Could you check a few things on this model? Use its own coordinates, in mm. A direction names the side the tool comes from. Give positions to 0.01 mm unless a question says otherwise; leave off trailing zeros. Order: outer loops, then holes, each group sorted by start corner. A loop starts at its lowest first (then second) coordinate and runs counter-clockwise, first axis right, second up. Notation, with made-up numbers: (16.25, 74) -> (58.25, 74) arc R21 ccw to (58.25, 107) -> close; hole circle Ø1 at (17.25, -15.5). An arc over 180 degrees is marked (long way). Write each question's results on one line, items separated by ' | '.
```python
from build123d import *

# Parameters (mm, degrees)
SKETCH3_R          = 1.4478
CUT_EXTRUDE1_DEPTH = 1.016
FILLET1_R          = 0.508
FILLET3_R          = 0.762


with BuildPart() as part:
    # Sketch2 → Revolve1 (revolve)
    with BuildSketch(Plane.XY):
        with BuildLine():
            Line((0, 0), (-4.7625, 0))
            Line((-4.7625, 0), (-4.7625, 0.254))
            ThreePointArc((-4.7625, 0.254), (-3.827073968, 1.183884704), (-2.5527, 1.524))
            Line((-2.5527, 1.524), (0, 1.524))
            Line((0, 1.524), (0, 0))
        make_face()
    revolve(axis=Axis((0, -4.155418325, 0), (0, 1, 0)))

    # Sketch3 → Cut-Extrude1 (cut)
    with BuildSketch(Plane(origin=(0, 1.524, 0), x_dir=(1, 0, 0), z_dir=(0, 1, 0))):
        Circle(SKETCH3_R)
    extrude(amount=-CUT_EXTRUDE1_DEPTH, mode=Mode.SUBTRACT)

    # Fillet1
    fillet1_edges = [part.edges().sort_by_distance(p)[0] for p in [
        (-1.4478, 1.524, 0),
    ]]
    fillet(fillet1_edges, radius=FILLET1_R)

    # Sketch5 → Revolve3 (revolve)
    with BuildSketch(Plane.XY):
        Polygon((0, 0), (-2.38125, 0), (-2.38125, -4.7625), (-3.175, -4.7625), (-3.175, -7.9375), (-1.4478, -7.9375), (-1.4478, -5.3975), (0, -5.3975), align=None)
    revolve(axis=Axis((0, 0, 0), (0, 1, 0)))

    # Fillet3
    fillet3_edges = [part.edges().sort_by_distance(p)[0] for p in [
        (3.175, -7.9375, 0),
    ]]
    fillet(fillet3_edges, radius=FILLET3_R)


solid = part.part
```
Q1. I'm going to push flat-ended pins straight in: pin 1 Ø3 at (x, y) = (2, -7) entering from -Z; pin 2 Ø5 at (x, y) = (-2.5, -6) entering from +Z (3 decimals); pin 3 Ø2 at (y, z) = (-5, 2) entering from -X; pin 4 Ø1.5 at (x, y) = (-3.5, -2) entering from +Z. Where does each tip first touch, or does it pass through?
Here are the results:
pin 1: stops at z = -3.14 | pin 2: stops at z = 3.175 | pin 3: stops at x = -3.01 | pin 4: passes through
Q2. Thinking about a two-plate mould opening in Z: for faces 5 (the cylindrical face through (0.314, -6.65, -1.413)), 6 (the cylindrical face through (1.89, -2.41, -1.45)), 7 (the cylindrical face through (-0.314, 0.766, 1.413)), 8 (the flat face through (0, -7.938, -2)), which applies, +Z half, -Z half, draft (parallel to the pull), parting line (faces both ways), or undercut?
Here are the results:
face 5: undercut | face 6: parting line | face 7: undercut | face 8: draft
Q3. For faces 1 (the flat face through (1, 1.524, -2)), 2 (the flat face through (0, 0.508, 0)), 3 (the flat face through (0, -5.398, 0)), 4 (the flat face through (2, 0, -2)), which set-ups out of +Z, -Z, +X, -X, +Y, -Y let a thin tool reach every point of the face, with its end or its side?
Here are the results:
face 1: +Z, -Z, +X, -X, +Y | face 2: +Y | face 3: -Y | face 4: none
Q4. Suppose I cut it at A-A on y = -4.5. Please give me the cut outline in (x, z), and give its area (3 significant figures).
Here are the results:
outline: circle Ø4.76 at (0, 0) | area: 17.8 mm²
Q5. I need wall thicknesses on line 1 along Z through (x, y) = (0, -6.7) (3 decimals); line 2 along Z through (x, y) = (0, 0.7); line 3 along X through (y, z) = (1.25, 1). Which ranges of each line are inside material? Lowest first, please.
Here are the results:
line 1: z = -3.175 to -1.448, 1.448 to 3.175 | line 2: z = -4.43 to -1.45, 1.45 to 4.43 | line 3: x = -3.57 to -1.12, 1.12 to 3.57
